```python
from build123d import *

# Parameters (mm, degrees)
F0_W            = 357
F0_H            = 3
F1_DEPTH        = 3
F2_W            = 6
F2_H            = 6
F3_DEPTH        = 15
F4_W            = 6
F4_H            = 6
F5_DEPTH        = 15
F6_R            = 2.36
F7_DEPTH        = 14
F8_R            = 2.565
F9_DEPTH        = 308
F10_R           = 2.36
F11_DEPTH       = 28
F12_DEPTH       = 15.1
F13_R           = 3.5
F14_DEPTH       = 20
F15_2_S5_R      = 2.36
F15_2_T6_DEPTH  = 5
F15_2_S11_R     = 2.36
F15_2_T12_DEPTH = 5
F17_DEPTH       = 5.8
F18_R           = 0.5


# Not quite as in the source:
# - a fillet or chamfer that OpenCascade refuses, or shapes differently, is made with other operations: its cross-section is extruded or revolved along the edge and cut away or added


with BuildPart() as f1:
    # F0 (on Front) → F1 (new body, symmetric)
    with BuildSketch(Plane.XZ):
        with Locations((178.5, 1.5)):
            Rectangle(F0_W, F0_H)
    extrude(amount=F1_DEPTH, both=True)


with BuildPart() as f3:
    # F2 (on face) → F3 (new body)
    with BuildSketch(Plane.YZ.offset(357)):
        with Locations((0, 6)):
            Rectangle(F2_W, F2_H)
    extrude(amount=-F3_DEPTH)



with BuildPart() as f5:
    # F4 (on face) → F5 (new body)
    with BuildSketch(Plane(origin=(0, 0, 0), x_dir=(0, -1, 0), z_dir=(-1, 0, 0))):
        with Locations((0, 6)):
            Rectangle(F4_W, F4_H)
    extrude(amount=-F5_DEPTH)



with BuildPart() as f7:
    # F6 (on face) → F7 (new body)
    with BuildSketch(Plane(origin=(342, 0, 0), x_dir=(0, -1, 0), z_dir=(-1, 0, 0))):
        with Locations((0, 6)):
            Circle(F6_R)
    extrude(amount=F7_DEPTH)

    # F8 (on face) → F9 (join)
    with BuildSketch(Plane(origin=(328, 0, 0), x_dir=(0, -1, 0), z_dir=(-1, 0, 0))):
        with Locations((0, 6)):
            Circle(F8_R)
    extrude(amount=F9_DEPTH)


with BuildPart() as f5_1:
    add(f5.part)

    add(f7.part)  # F11 merges F7
    # F10 (on face) → F11 (join)
    with BuildSketch(Plane(origin=(20, 0, 0), x_dir=(0, -1, 0), z_dir=(-1, 0, 0))):
        with Locations((0, 6)):
            Circle(F10_R)
    extrude(amount=F11_DEPTH)


with BuildPart() as f3_1:
    add(f3.part)

    add(f5_1.part)  # F12 merges F5
    # F6 (on face) → F12 (join)
    with BuildSketch(Plane(origin=(342, 0, 0), x_dir=(0, -1, 0), z_dir=(-1, 0, 0))):
        with Locations((0, 6)):
            Circle(F6_R)
    extrude(amount=-F12_DEPTH)

    # F15#2: chamfer of 1 on 2 edges, made by hand


with BuildPart() as f14:
    # F13 (on face) → F14 (new body)
    with BuildSketch(Plane(origin=(-8, 0, 0), x_dir=(0, -1, 0), z_dir=(-1, 0, 0))):
        with Locations((0, 6)):
            Circle(F13_R)
    extrude(amount=F14_DEPTH)

    # F15: chamfer of 1 on 1 edges, made by hand

    # F15_s1 → F15_t2 (revolve, cut)
    with BuildSketch(Plane.XY.offset(6)):
        Polygon((-9, -3.5), (-8, -2.5), (-8, -3.5), align=None)
    revolve(axis=Axis((-8, 0, 6), (-1, 0, 0)), mode=Mode.SUBTRACT)

    # F16 (on face) → F17 (cut)
    with BuildSketch(Plane(origin=(-28, 0, 0), x_dir=(0, -1, 0), z_dir=(-1, 0, 0))):
        Polygon((0, 3.6905989232), (2, 4.8452994616), (2, 7.1547005384), (0, 8.3094010768), (-2, 7.1547005384), (-2, 4.8452994616), align=None)
    extrude(amount=-F17_DEPTH, mode=Mode.SUBTRACT)

    # F18
    f18_edges = [f14.edges().sort_by_distance(p)[0] for p in [
        (-22.2, 1, 4.267949),
        (-22.2, -1, 4.267949),
        (-22.2, -2, 6),
        (-22.2, -1, 7.732051),
        (-22.2, 1, 7.732051),
        (-22.2, 2, 6),
    ]]
    fillet(f18_edges, radius=F18_R)


with BuildPart() as f15_2_tool2:
    # F15_2_s3 → F15_2_t4 (revolve)
    with BuildSketch(Plane.XY.offset(6)):
        Polygon((21, -2.565), (20, -1.565), (20, -2.565), align=None)
    revolve(axis=Axis((20, 0, 6), (-1, 0, 0)))

    # F15_2_s5 → F15_2_t6 (cut, symmetric)
    with BuildSketch(Plane.YZ.offset(20.5)):
        with Locations((0, 6)):
            Circle(F15_2_S5_R)
    extrude(amount=F15_2_T6_DEPTH, both=True, mode=Mode.SUBTRACT)


with BuildPart() as f3_2:
    add(f3_1.part)

    # F15_2_t1: cut F15_2_tool2
    add(f15_2_tool2.part, mode=Mode.SUBTRACT)


with BuildPart() as f15_2_tool8:
    # F15_2_s9 → F15_2_t10 (revolve)
    with BuildSketch(Plane.XY.offset(6)):
        Polygon((328, -1.565), (327, -2.565), (328, -2.565), align=None)
    revolve(axis=Axis((328, 0, 6), (-1, 0, 0)))

    # F15_2_s11 → F15_2_t12 (cut, symmetric)
    with BuildSketch(Plane.YZ.offset(327.5)):
        with Locations((0, 6)):
            Circle(F15_2_S11_R)
    extrude(amount=F15_2_T12_DEPTH, both=True, mode=Mode.SUBTRACT)


with BuildPart() as f3_3:
    add(f3_2.part)

    # F15_2_t7: cut F15_2_tool8
    add(f15_2_tool8.part, mode=Mode.SUBTRACT)


with BuildPart() as f1_1:
    add(f1.part)

    # F19: union F3, F14
    add(f3_3.part)
    add(f14.part)


solid = f1_1.part
```
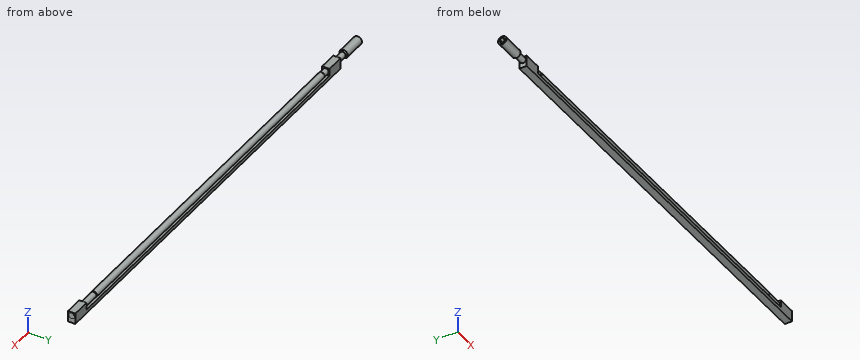
Source: CAD feature listing. Evaluate the final solid. Frame: model axes, mm. Round coordinates to 2 decimals unless told otherwise and drop trailing zeros. Loops run counter-clockwise (first coordinate to the right, second up) from the corner with the lowest first, then second, coordinate; pieces in that order, holes last.
(1) Material intervals for probe 1 along Z at (x, y) = (299, -0.75); probe 2 along X at (y, z) = (-2.25, 3.5); probe 3 along X at (y, z) = (1.75, 1.25), sorted ascending.
From the geometry:
probe 1: z = 0 to 3, 3.55 to 8.45
probe 2: x = -28 to -8.86, 0 to 15, 342 to 357
probe 3: x = 0 to 357
(2) Section query A-A (x = 88). Output: boundary loops of the cut face in (y, z) (3 decimals).
From the geometry:
outline: (-3, 0) - (3, 0) - (3, 3) - (-3, 3) - close; circle Ø5.13 at (0, 6)
(3) Contact query for flat-ended pins moving along their axis: pin 1 Ø4 at (x, z) = (264.5, 7) entering from +Y (3 decimals); pin 2 Ø4.5 at (x, z) = (95.5, 3.5) entering from -Y. Output: stop coordinate, or through.
From the geometry:
pin 1: stops at y = 2.565
pin 2: stops at y = -3
